The listing builds one solid part. Answer for the finished solid, in the listing's coordinates (mm). A direction names the side the tool comes from. Give positions to 0.01 mm unless a question says otherwise; leave off trailing zeros. Order: outer loops, then holes, each group sorted by start corner. A loop starts at its lowest first (then second) coordinate and runs counter-clockwise, first axis right, second up. Notation, with made-up numbers: (64.5, 87) - (76.5, 87) arc R23 cw to (76.5, 108) - close; hole circle Ø3 at (23.5, 33.5). An arc over 180 degrees is marked (long way). Answer in a Markdown table with one row per item.
from build123d import *

# Parameters (mm, degrees)
F0_R     = 0.75
F1_DEPTH = 2
F2_DEPTH = 5


with BuildPart() as f1:
    # F0 (on Top) → F1 (new body)
    with BuildSketch(Plane.XY):
        with BuildLine():
            ThreePointArc((12.5, 0), (8.8388347648, 8.8388347648), (0, 12.5))
            ThreePointArc((0, 12.5), (-8.8388347648, -8.8388347648), (12.5, 0))
        make_face()
        with Locations((-8.6602540378, -5)):
            Circle(F0_R, mode=Mode.SUBTRACT)
        with Locations((-5.4126587737, -3.125)):
            Circle(F0_R, mode=Mode.SUBTRACT)
        with Locations((5.4126587737, -3.125)):
            Circle(F0_R, mode=Mode.SUBTRACT)
        with Locations((8.6602540378, -5)):
            Circle(F0_R, mode=Mode.SUBTRACT)
        with BuildLine():
            ThreePointArc((4, 0), (-2.8284271247, -2.8284271247), (0, 4))
            ThreePointArc((0, 4), (2.8284271247, 2.8284271247), (4, 0))
        make_face(mode=Mode.SUBTRACT)
        with BuildLine():
            ThreePointArc((0.75, 6.25), (0.5303300859, 5.7196699141), (0, 5.5))
            ThreePointArc((0, 5.5), (-0.75, 6.25), (0, 7))
            ThreePointArc((0, 7), (0.5303300859, 6.7803300859), (0.75, 6.25))
        make_face(mode=Mode.SUBTRACT)
        with BuildLine():
            ThreePointArc((0.75, 10), (0.5303300859, 9.4696699141), (0, 9.25))
            ThreePointArc((0, 9.25), (-0.75, 10), (0, 10.75))
            ThreePointArc((0, 10.75), (0.5303300859, 10.5303300859), (0.75, 10))
        make_face(mode=Mode.SUBTRACT)
    extrude(amount=F1_DEPTH)

    # F0 (on Top) → F2 (join)
    with BuildSketch(Plane.XY):
        with BuildLine():
            ThreePointArc((4, 0), (2.8284271247, 2.8284271247), (0, 4))
            ThreePointArc((0, 4), (-2.8284271247, -2.8284271247), (4, 0))
        make_face()
        with BuildLine():
            ThreePointArc((1.5612494996, 1.25), (1.8871273141, 0.6623824427), (2, 0))
            ThreePointArc((2, 0), (1.8871273141, -0.6623824427), (1.5612494996, -1.25))
            ThreePointArc((1.5612494996, -1.25), (0, -2), (-1.5612494996, -1.25))
            ThreePointArc((-1.5612494996, -1.25), (-2, 0), (-1.5612494996, 1.25))
            ThreePointArc((-1.5612494996, 1.25), (-0.8660254038, 1.8027756377), (0, 2))
            ThreePointArc((0, 2), (0.8660254038, 1.8027756377), (1.5612494996, 1.25))
        make_face(mode=Mode.SUBTRACT)
        with BuildLine():
            Line((0, 1.25), (1.5612494996, 1.25))
            ThreePointArc((1.5612494996, 1.25), (0.8660254038, 1.8027756377), (0, 2))
            Line((0, 2), (0, 1.25))
        make_face()
        with BuildLine():
            Line((0, 1.25), (0, 2))
            ThreePointArc((0, 2), (-0.8660254038, 1.8027756377), (-1.5612494996, 1.25))
            Line((-1.5612494996, 1.25), (0, 1.25))
        make_face()
        with BuildLine():
            ThreePointArc((-1.5612494996, -1.25), (0, -2), (1.5612494996, -1.25))
            Line((1.5612494996, -1.25), (-1.5612494996, -1.25))
        make_face()
    extrude(amount=F2_DEPTH)


solid = f1.part
Item 1: Determine the mould class of faces 3 (the face through (9.35, -5.29, 0.99)), 4 (the face through (4.663, -3.092, 0.986)), 5 (the face through (-3, 3, 2)) for opening direction X: pulls with the +X half, pulls with the -X half, needs draft (parallel to the pull), parting line crosses it, or undercut.
Answer block:
| item | result |
|---|---|
| face 3 | undercut |
| face 4 | undercut |
| face 5 | needs draft |
Item 2: Find section B-B on z = 1.3. Write down the section's boundary in (x, y) (3 decimals), then the cut area to 3 significant figures.
Answer block:
| item | result |
|---|---|
| outline | circle Ø25 at (0, 0); hole circle Ø1.5 at (-8.66, -5); hole circle Ø1.5 at (-5.413, -3.125); hole (-1.561, -1.25) - (1.561, -1.25) arc R2 ccw to (1.561, 1.25) - (-1.561, 1.25) arc R2 ccw to start; hole circle Ø1.5 at (0, 6.25); hole circle Ø1.5 at (0, 10); hole circle Ø1.5 at (5.413, -3.125); hole circle Ø1.5 at (8.66, -5) |
| area | 471 mm² |
Item 3: Find section C-C on y = 2.5. Write down the section's boundary in (x, z), then the cut area to 3 significant figures.
Answer block:
| item | result |
|---|---|
| outline | (-12.25, 0) - (12.25, 0) - (12.25, 2) - (3.12, 2) - (3.12, 5) - (-3.12, 5) - (-3.12, 2) - (-12.25, 2) - close |
| area | 67.7 mm² |
Item 4: Find section A-A on y = -2.75. Write down the section's boundary in (x, z), then the cut area to 3 significant figures.
Answer block:
| item | result |
|---|---|
| outline | (-12.19, 0) - (-6.06, 0) - (-6.06, 2) - (-12.19, 2) - close; (-4.76, 0) - (4.76, 0) - (4.76, 2) - (2.9, 2) - (2.9, 5) - (-2.9, 5) - (-2.9, 2) - (-4.76, 2) - close; (6.06, 0) - (12.19, 0) - (12.19, 2) - (6.06, 2) - close |
| area | 61.0 mm² |
Item 5: Which of the six approach directions +Z, -Z, +X, -X, +Y, -Y give full straight-line access (tool end or side, diameter ignored) to faces 1 (the face through (-2, 0, 2)), 2 (the face through (0, -2, 5))?
Answer block:
| item | result |
|---|---|
| face 1 | +Z, -Z |
| face 2 | +Z, +X, -X, +Y, -Y |
Item 6: Consider line 1 (Z direction, x = 5.5, y = -8); line 2 (Y direction, x = -0.25, z = 1.8); line 3 (Y direction, x = 1.75, z = 1.15). Determine where each line is inside the solid, lowest interval first.
Answer block:
| item | result |
|---|---|
| line 1 | 0 to 2 |
| line 2 | -12.5 to -1.25, 1.25 to 5.54, 6.96 to 9.29, 10.71 to 12.5 |
| line 3 | -12.38 to -0.97, 0.97 to 12.38 |
Item 7: Find section D-D on x = 2.75. Write down the section's boundary in (y, z).
Answer block:
| item | result |
|---|---|
| outline | (-12.19, 0) - (12.19, 0) - (12.19, 2) - (2.9, 2) - (2.9, 5) - (-2.9, 5) - (-2.9, 2) - (-12.19, 2) - close |
Item 8: Each of these flat-tipped pins is pushed along its axis until it touches: P1, Ø0.9, axis at x = 5.41, y = -3.12, coming from the -Z side; P2, Ø3, axis at x = 8, z = 2.5, coming from the -Y side; P3, Ø1, axis at x = 7, y = -2, coming from the +Z side; P4, Ø3, axis at y = 5, z = 3, coming from the -X side. Where does it stop, or does it pass through?
Answer block:
| item | result |
|---|---|
| P1 | through |
| P2 | y = -10.62 |
| P3 | z = 2 |
| P4 | x = -11.88 |
